from build123d import *

# Parameters (mm, degrees)
SKETCH1_R           = 127
BOSS_EXTRUDE1_DEPTH = 25.4
SKETCH2_R           = 9.54156828
BOSS_EXTRUDE2_DEPTH = 6.35
CIRPATTERN1_COUNT   = 8
SKETCH3_R           = 50.944165106
BOSS_EXTRUDE3_DEPTH = 19.05
SKETCH4_R           = 25.4
CUT_EXTRUDE1_DEPTH  = 132.334


with BuildPart() as part:
    # Sketch1 → Boss-Extrude1 (new body)
    with BuildSketch(Plane(origin=(0, 0, 0), x_dir=(0, 0, -1), z_dir=(1, 0, 0))):
        Circle(SKETCH1_R)
    extrude(amount=BOSS_EXTRUDE1_DEPTH)

    # Sketch2 → Boss-Extrude2 (add)
    with BuildSketch(Plane(origin=(25.4, 0, 0), x_dir=(0, 0, -1), z_dir=(1, 0, 0))):
        with Locations((0, 100.208781769)):
            Circle(SKETCH2_R)
    boss_extrude2 = extrude(amount=BOSS_EXTRUDE2_DEPTH)

    # CirPattern1: Boss-Extrude2 ×8 about axis
    cirpattern1_axis = Axis((0, -0.568847983, 0), (1, 0, 0))
    for i in range(1, CIRPATTERN1_COUNT):
        add(boss_extrude2.rotate(cirpattern1_axis, i * 360 / CIRPATTERN1_COUNT))

    # Sketch3 → Boss-Extrude3 (add)
    with BuildSketch(Plane(origin=(25.4, 0, 0), x_dir=(0, 0, -1), z_dir=(1, 0, 0))):
        with Locations(Location((0, 0, 0), (0, 0, 180))):
            Circle(SKETCH3_R)
    extrude(amount=BOSS_EXTRUDE3_DEPTH)

    # Sketch4 → Cut-Extrude1 (cut)
    with BuildSketch(Plane(origin=(44.45, 0, 0), x_dir=(0, 0, -1), z_dir=(1, 0, 0))):
        Circle(SKETCH4_R)
    extrude(amount=-CUT_EXTRUDE1_DEPTH, mode=Mode.SUBTRACT)


solid = part.part
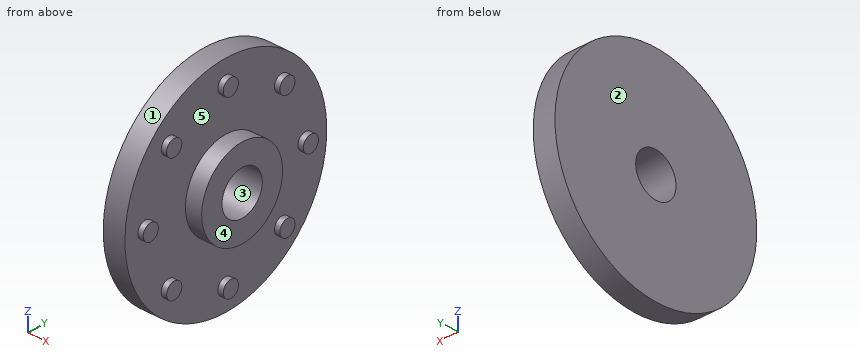
Work out the finished part from the listing and answer in its coordinate system (mm). Face numbers are marked on the shaded views. A direction names the side the tool comes from. Round coordinates to 2 decimals unless told otherwise and drop trailing zeros. Loops run counter-clockwise (first coordinate to the right, second up) from the corner with the lowest first, then second, coordinate; pieces in that order, holes last. Notation, with made-up numbers: M 64,79 L 122,79 A21 ccw 122,95 Z; hole C -36.75,63 d6. An arc over 180 degrees is marked long. One line per question, with ' | ' between items. Start each with the question number.
(1) A cutting plane is placed at B-B on y = 0. Write down the section's boundary in (x, z).
(2) A cutting plane is placed at C-C on z = -75. Write down the section's boundary in (x, y).
(3) Flat-ended cylindrical pins translate along their axes: pin 1 Ø5.5 at (y, z) = (-73, 70.5) entering from +X; pin 2 Ø8 at (y, z) = (83.5, 2.5) entering from +X; pin 3 Ø3 at (x, y) = (7.5, -66) entering from +Z. Find the tip coordinate at first contact, or state that the pin passes through.
(4) A tool of negligible diameter and unlimited length cuts with its end or side. For the marked faces 4 and 5, from which of +Z, -Z, +X, -X, +Y, -Y can it reach the whole face along a straight path? Write none if from no direction.
(5) For a pull along Y with two mould halves and no side action, classify the marked faces 1, 2 and 3 as released by +Y, released by -Y, zero draft, split by the parting line, or undercut.
(6) A cutting plane is placed at D-D on x = 6. Write down the section's boundary in (y, z).
(7) Find the intervals of material crossed by line 1 (Y direction, x = 25, z = 0); line 2 (Z direction, x = 20, y = 1); line 3 (X direction, y = -53.5, z = -23), in increasing order.
(8) A cutting plane is placed at A-A on z = 0. Write down the section's boundary in (x, y).
Geometry check:
1) outline: M 0,-127 L 25.4,-127 L 25.4,-110.3 L 31.75,-110.3 L 31.75,-91.25 L 25.4,-91.25 L 25.4,-50.94 L 44.45,-50.94 L 44.45,-25.4 L 0,-25.4 Z; M 0,25.4 L 44.45,25.4 L 44.45,50.94 L 25.4,50.94 L 25.4,91.25 L 31.75,91.25 L 31.75,110.3 L 25.4,110.3 L 25.4,127 L 0,127 Z
2) outline: M 0,-102.49 L 25.4,-102.49 L 25.4,-80.61 L 31.75,-80.61 L 31.75,-63.05 L 25.4,-63.05 L 25.4,61.91 L 31.75,61.91 L 31.75,79.47 L 25.4,79.47 L 25.4,102.49 L 0,102.49 Z
3) pin 1: stops at x = 31.75 | pin 2: stops at x = 25.4 | pin 3: stops at z = 109.4
4) face 4: +Z, -Z, +X, +Y, -Y | face 5: +X
5) face 1: split by the parting line | face 2: zero draft | face 3: undercut
6) outline: C 0,0 d254; hole C 0,0 d50.8
7) line 1: y = -127 to -25.4, 25.4 to 127 | line 2: z = -127 to -25.38, 25.38 to 127 | line 3: x = 0 to 25.4
8) outline: M 0,-127 L 25.4,-127 L 25.4,-110.89 L 31.75,-110.89 L 31.75,-91.8 L 25.4,-91.8 L 25.4,-50.94 L 44.45,-50.94 L 44.45,-25.4 L 0,-25.4 Z; M 0,25.4 L 44.45,25.4 L 44.45,50.94 L 25.4,50.94 L 25.4,90.67 L 31.75,90.67 L 31.75,109.75 L 25.4,109.75 L 25.4,127 L 0,127 Z
